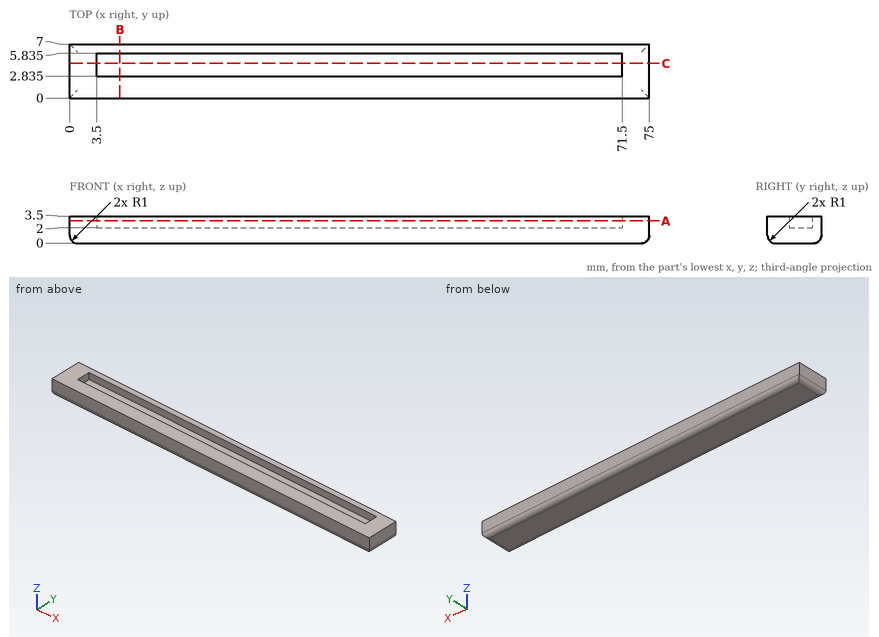
Geometry check sheet. Reference: drawing and pictorial views, mm from the part's lowest x, y, z. Coordinates: 2 decimals unless noted, no trailing zeros. Loops run counter-clockwise (first coordinate to the right, second up) from the corner with the lowest first, then second, coordinate; pieces in that order, holes last.
1) Material ranges on probe 1 along Y at (x, z) = (30, 3.4) (1 decimal); probe 2 along X at (y, z) = (3, 2.7); probe 3 along Z at (x, y) = (42, 4.75), recorded low to high.
2) Sectioned sample at B-B (x = 6.5). Record the boundary of the cut face in (y, z) (1 decimal).
3) Sectioned sample at C-C (y = 4.5). Record the boundary of the cut face in (x, z).
4) Sectioned sample at A-A (z = 2.9). Record the boundary of the cut face in (x, y) (1 decimal).
5) Gauge pin test, flat end, axial feed: pin 1 (2.5 mm diameter, centred on x = 29.5, y = 4.5, fed in from +Z). Record the tip position at first contact, or that the pin passes through.
Check sheet entries:
1. probe 1: y = 0 to 2.8, 5.8 to 7
1. probe 2: x = 0 to 3.5, 71.5 to 75
1. probe 3: z = 0 to 2
2. outline: (0, 1) arc R1 ccw to (1, 0) - (6, 0) arc R1 ccw to (7, 1) - (7, 3.5) - (5.8, 3.5) - (5.8, 2) - (2.8, 2) - (2.8, 3.5) - (0, 3.5) - close
3. outline: (0, 1) arc R1 ccw to (1, 0) - (74, 0) arc R1 ccw to (75, 1) - (75, 3.5) - (71.5, 3.5) - (71.5, 2) - (3.5, 2) - (3.5, 3.5) - (0, 3.5) - close
4. outline: (0, 0) - (75, 0) - (75, 7) - (0, 7) - close; hole (3.5, 2.8) - (71.5, 2.8) - (71.5, 5.8) - (3.5, 5.8) - close
5. pin 1: stops at z = 2
